```python
from build123d import *

# Parameters (mm, degrees)
F0_R     = 50
F1_DEPTH = 10
F2_R     = 5
F3_R     = 4.99999


# Not quite as in the source:
# - a fillet or chamfer is up to 0.001 mm smaller than in the source, because OpenCascade refuses the exact size


with BuildPart() as f1:
    # F0 (on Top) → F1 (new body)
    with BuildSketch(Plane.XY):
        Circle(F0_R)
    extrude(amount=F1_DEPTH)

    # F2
    f2_edges = [f1.edges().sort_by_distance(p)[0] for p in [
        (-50, 0, 10),
    ]]
    fillet(f2_edges, radius=F2_R)

    # F3 (radius 5 in the source; OpenCascade refuses exactly that, so slightly less here)
    f3_edges = [f1.edges().sort_by_distance(p)[0] for p in [
        (-50, 0, 0),
    ]]
    fillet(f3_edges, radius=F3_R)


solid = f1.part
```
Verification items for the finished model (mm, model axes). Coordinates: 2 decimals unless noted, no trailing zeros. Loops run counter-clockwise (first coordinate to the right, second up) from the corner with the lowest first, then second, coordinate; pieces in that order, holes last. Notation, with made-up numbers: (-25, 22) -> (3, 22) arc R20 ccw to (3, 42) -> close; hole circle Ø9 at (-34.5, 49). An arc over 180 degrees is marked (long way). Answer in a Markdown table with one row per item.
1) Section check C-C (z = 1.5). Record the cut outline in (x, y), and give its area (3 significant figures).
The answers:
| item | result |
|---|---|
| outline | circle Ø97.14 at (0, 0) |
| area | 7,410 mm2 |
2) Depth check by flat-ended pin: P1, Ø1, axis at y = 28.5, z = 8, coming from the -X side; P2, Ø1.5, axis at x = -6, z = 8, coming from the +Y side; P3, Ø1, axis at x = -18.5, z = 8.5, coming from the +Y side. Enter the tip coordinate at first touch or a pass-through.
The answers:
| item | result |
|---|---|
| P1 | stops at x = -40.41 |
| P2 | stops at y = 49.11 |
| P3 | stops at y = 45.42 |
3) Scan lines: line 1 along X through (y, z) = (16.5, 9.25); line 2 along X through (y, z) = (32, 8.5); line 3 along Y through (x, z) = (-23.5, 0.75). Record each from-to range of solid material in increasing order. Write a range as from..to.
The answers:
| item | result |
|---|---|
| line 1 | x = -44.68..44.68 |
| line 2 | x = -36.54..36.54 |
| line 3 | y = -41.43..41.43 |
